Can you work these out from the model? Positions are in its coordinate system, mm. A direction names the side the tool comes from. Give positions to 0.01 mm unless a question says otherwise; leave off trailing zeros. Write each loop counter-clockwise with the first axis right and the second up, starting at its lowest first coordinate (ties: lowest second). Pieces come first, ordered by that corner, then holes.
Autodesk Inventor part; units mm, degrees
ref_plane "YZ Plane" through (0, 0, 0) normal (1, 0, 0) x (0, 1, 0)
ref_plane "XZ Plane" through (0, 0, 0) normal (0, 1, 0) x (-1, 0, 0)
ref_plane "XY Plane" through (0, 0, 0) normal (0, 0, 1) x (1, 0, 0)
sketch "草圖1" plane through (0, 0, 0) normal (0, 0, 1) x (1, 0, 0)
  point P0 (0, 0)
sketch "草圖2" plane through (0, 0, 0) normal (0, 1, 0) x (-1, 0, 0)
  line L0 (6, 2.5) -> (-6, 2.5)
  line L1 (-6, 2.5) -> (-6, -2.5)
  line L2 (-6, -2.5) -> (6, -2.5)
  line L3 (6, -2.5) -> (6, 2.5)
  line L4 (6, 2.5) -> (-6, -2.5) construction
  line L5 (-6, 2.5) -> (6, -2.5) construction
  point P0 (0, 0)
  dimension "d0" = 5
  dimension "d1" = 12
extrude "擠出1" add sketch "草圖2" along normal blind 25
sketch "草圖3" plane through (-6, 0, 2.5) normal (0, 0, 1) x (1, 0, 0)
  circle A0 centre (6, 10) radius 2.6
  circle A1 centre (6, 20) radius 2.6
  line L0 (0, 0) -> (12, 0)
  point P0 (6, 0)
  point P1 (6, 0)
  dimension "d4" = 5.2
  dimension "d5" = 5.2
  dimension "d6" = 10
  dimension "d7" = 10
extrude "擠出2" cut sketch "草圖3" against normal blind 5.2
sketch "草圖4" plane through (0, 0, 0) normal (0, -1, 0) x (1, 0, 0)
  line L0 (-10, -10) -> (10, -10)
  line L1 (10, -10) -> (10, 10)
  line L2 (10, 10) -> (-10, 10)
  line L3 (-10, 10) -> (-10, -10)
  line L4 (-10, -10) -> (10, 10) construction
  line L5 (10, -10) -> (-10, 10) construction
  point P0 (0, 0)
  dimension "d10" = 20
  dimension "d11" = 20
extrude "擠出3" add sketch "草圖4" along normal blind 2
sketch "草圖5" plane through (0, -2, 0) normal (0, -1, 0) x (1, 0, 0)
  line L0 (-0.95, -1.15) -> (0.95, -1.15)
  line L1 (0.95, -1.15) -> (0.95, 1.15)
  line L2 (0.95, 1.15) -> (-0.95, 1.15)
  line L3 (-0.95, 1.15) -> (-0.95, -1.15)
  line L4 (-0.95, -1.15) -> (0.95, 1.15) construction
  line L5 (0.95, -1.15) -> (-0.95, 1.15) construction
  point P0 (0, 0)
  dimension "d14" = 1.9
  dimension "d15" = 2.3
extrude "擠出4" add sketch "草圖5" along normal blind 5
sketch "草圖6" plane through (0, -2, 0) normal (0, -1, 0) x (1, 0, 0)
  line L0 (-4, -3) -> (4, -3)
  line L1 (4, -3) -> (4, 3)
  line L2 (4, 3) -> (-4, 3)
  line L3 (-4, 3) -> (-4, -3)
  line L4 (-4, -3) -> (4, 3) construction
  line L5 (4, -3) -> (-4, 3) construction
  line L6 (-5, -3.75) -> (5, -3.75)
  line L7 (5, -3.75) -> (5, 3.75)
  line L8 (5, 3.75) -> (-5, 3.75)
  line L9 (-5, 3.75) -> (-5, -3.75)
  line L10 (-5, -3.75) -> (5, 3.75) construction
  line L11 (5, -3.75) -> (-5, 3.75) construction
  point P0 (0, 0)
  dimension "d18" = 6
  dimension "d19" = 8
  dimension "d20" = 10
extrude "擠出5" add sketch "草圖6" along normal blind 5
sketch "草圖7" plane through (5, -2, 3.75) normal (1, 0, 0) x (0, 0, -1)
  line L0 (7.5, -5) -> (0, -5)
  line L1 (2.3009, -5) -> (5.1991, -5) construction
  line L2 (2.75, -4.5509) -> (4.75, -4.5509)
  line L3 (4.75, -5.4491) -> (2.75, -5.4491)
  arc A0 (2.75, -4.5509) -> (2.75, -5.4491) centre (2.75, -5) ccw
  arc A1 (4.75, -5.4491) -> (4.75, -4.5509) centre (4.75, -5) ccw
  line L4 (-6.25, 0) -> (13.75, 0)
  line L5 (3.75, 0) -> (3.75, -5)
  line L6 (0, 0) -> (0, -5)
  point P0 (3.75, 2)
  point P1 (5.1991, -5)
  dimension "d23" = 2
  dimension "d26" = 3.75
extrude "擠出6" cut sketch "草圖7" against normal blind 2 contours L0 L5 L2 A1 | L0 A0 L2 L5
sketch "草圖8" plane through (0, 0, 0) normal (0, 1, 0) x (1, 0, 0)
  line L0 (10, 10) -> (10, -10)
  line L1 (7, -4.5) -> (10, -4.5)
  line L2 (10, -4.5) -> (10, -2)
  line L3 (10, -2) -> (7, -2)
  line L4 (7, -2) -> (7, -4.5)
  line L5 (7, 2) -> (10, 2)
  line L6 (10, 2) -> (10, 4.5)
  line L7 (10, 4.5) -> (7, 4.5)
  line L8 (7, 4.5) -> (7, 2)
  point P0 (0, 0)
  point P1 (10, 0)
  point P2 (10, 0)
  dimension "d27" = 3
  dimension "d28" = 2.5
  dimension "d29" = 2.5
  dimension "d30" = 2
  dimension "d31" = 2
extrude "擠出7" cut sketch "草圖8" against normal blind 2
sketch "草圖9" plane through (0, -7, 0) normal (0, -1, 0) x (1, 0, 0)
  line L0 (6.5, 5) -> (-6.5, 5)
  line L1 (-6.5, 5) -> (-6.5, -5)
  line L2 (-6.5, -5) -> (6.5, -5)
  line L3 (6.5, -5) -> (6.5, 5)
  line L4 (6.5, 5) -> (-6.5, -5) construction
  line L5 (-6.5, 5) -> (6.5, -5) construction
  point P0 (0, 0)
  dimension "d34" = 10
  dimension "d35" = 13
extrude "擠出8" add sketch "草圖9" along normal blind 0.5
sketch "草圖10" plane through (0, -7.5, 0) normal (0, -1, 0) x (1, 0, 0)
  line L0 (-4, 3) -> (-4, -3)
  line L1 (4, 3) -> (-4, 3)
  line L2 (-4, 3) -> (-4, -3)
  line L3 (-4, -3) -> (4, -3)
  line L4 (4, -3) -> (4, 3)
  line L5 (4, 3) -> (-4, -3) construction
  line L6 (-4, 3) -> (4, -3) construction
  point P0 (0, 0)
extrude "擠出9" cut sketch "草圖10" against normal blind 5
sketch "草圖11" plane through (0, -2.5, 0) normal (0, -1, 0) x (1, 0, 0)
  line L0 (0.95, -1.15) -> (-0.95, -1.15)
  line L1 (0.95, 1.15) -> (-0.95, 1.15)
  line L2 (-0.95, 1.15) -> (-0.95, -1.15)
  line L3 (-0.95, -1.15) -> (0.95, -1.15)
  line L4 (0.95, -1.15) -> (0.95, 1.15)
  line L5 (0.95, 1.15) -> (-0.95, -1.15) construction
  line L6 (-0.95, 1.15) -> (0.95, -1.15) construction
  point P0 (0, 0)
extrude "擠出10" add sketch "草圖11" along normal blind 5
equation "\"d8\" = d5"
properties part number "單線圈感測器上"
1) Suppose I cut it at D-D on z = 8.25. Write out the boundary of the cut face in (x, y), plus the area to 3 significant figures.
Values follow:
outline: (-10, -2) - (10, -2) - (10, 0) - (-10, 0) - close
area: 40.0 mm2
2) Suppose I cut it at A-A on y = 21. Write out the boundary of the cut face in (x, z).
Values follow:
outline: (-6, -2.5) - (-2.4, -2.5) - (-2.4, 2.5) - (-6, 2.5) - close; (2.4, -2.5) - (6, -2.5) - (6, 2.5) - (2.4, 2.5) - close
3) If we mould it in two halves opening along Z, with no side actions, what happens to faces 1 (the face through (-4, -5, 0)), 2 (the face through (-0.56, 7.46, 0.04)), 3 (the face through (9, -1, -4.5)), 4 (the face through (0, -1, 10))? For each: +Z half, -Z half, draft (parallel to the pull), parting line (faces both ways), or undercut.
Values follow:
face 1: undercut
face 2: draft
face 3: undercut
face 4: +Z half
4) Suppose I cut it at B-B on y = -3.5. Write out the boundary of the cut face in (x, z).
Values follow:
outline: (-5, -3.75) - (5, -3.75) - (5, 3.75) - (-5, 3.75) - close; (-0.95, -1.15) - (0.95, -1.15) - (0.95, 1.15) - (-0.95, 1.15) - close; hole (-4, -3) - (4, -3) - (4, 3) - (-4, 3) - close
5) Please list where these lines run through material, in increasing order: L1, parallel to Y at x = 0, z = 1.05; L2, parallel to Y at x = 0, z = -1.25; L3, parallel to X at y = -3, z = 0.25.
Values follow:
L1: y = -7.5 to 7.4, 12.6 to 17.4, 22.6 to 25
L2: y = -2 to 7.4, 12.6 to 17.4, 22.6 to 25
L3: x = -5 to -4, -0.95 to 0.95, 4 to 5
6) Suppose I cut it at C-C on x = 0. State how many separate pieces and enclosed holes the cut face has, plus the area to 3 significant figures.
Values follow:
separate pieces: 3
enclosed holes: 0
area: 135 mm2
7) For faces 5 (the face through (0.95, -5, 0)), 6 (the face through (9, -1, 2)), 7 (the face through (5, -4, 0)), which set-ups out of +Z, -Z, +X, -X, +Y, -Y let a thin tool reach every point of the face, with its end or its side?
Values follow:
face 5: -Y
face 6: +X, +Y, -Y
face 7: +Z, -Z, +X
8) For pin 1 Ø5.5 at (y, z) = (-5.5, 0.5) entering from +X; pin 2 Ø1.6 at (y, z) = (-4.5, -0.5) entering from +X; pin 3 Ø8.5 at (x, y) = (0, 20) entering from +Z, each with a flat end and sliding along its axis, tell me the tip position at first contact or that it passes through.
Values follow:
pin 1: stops at x = 6.5
pin 2: stops at x = 5
pin 3: stops at z = 2.5
